Verification items for the finished model (mm, model axes). A direction names the side the tool comes from. Give positions to 0.01 mm unless a question says otherwise; leave off trailing zeros. Loops run counter-clockwise (first coordinate to the right, second up) from the corner with the lowest first, then second, coordinate; pieces in that order, holes last. Notation, with made-up numbers: (55, 60.25) - (77, 60.25) arc R18 cw to (77, 83.25) - close; hole circle Ø2 at (69, 86.25). An arc over 180 degrees is marked (long way). One line per item, written item: value. Start each with the question number.
1. Sectioned sample at C-C (z = -107.5). Record the cut outline in (x, y).
2. Gauge pin test, flat ends, axial feed: pin 1 (2 mm diameter, centred on x = 3, y = 5, fed in from -Z); pin 2 (3 mm diameter, centred on y = 2, z = -12, fed in from -X); pin 3 (1.4 mm diameter, centred on x = 2.5, y = 5.5, fed in from +Z); pin 4 (0.8 mm diameter, centred on y = 5.5, z = -126, fed in from +X). Record the tip position at first contact, or that the pin passes through.
3. Sectioned sample at B-B (x = 5.5). Record the cut outline in (y, z), plus the area to 3 significant figures.
4. Sectioned sample at A-A (y = 6.25). Record the cut outline in (x, z).
5. Mould release check, pull along Z, two halves, no side actions. Record for faces 1 (the flat face through (2, 7.302, -64)), 2 (the flat face through (3.774, 3.6, -77.998)): pulls with the +Z half, pulls with the -Z half, needs draft (parallel to the pull), parting line crosses it, or undercut.
6. Access from +Z, -Z, +X, -X, +Y, -Y to the whole of each face (thin tool, end or side, straight path). Record for faces 3 (the flat face through (1.651, 4, 1)), 4 (the flat face through (1.651, 4, -127)), 5 (the flat face through (2, 0, -64)), 6 (the flat face through (2.164, 3.6, -15.384)), 7 (the flat face through (0, 4, -64)).
7. Scan lines: L1, parallel to X at y = 5.75, z = -63.5; L2, parallel to X at y = 6.25, z = -66.5. Record each from-to range of solid material in increasing order. Write a range as [from, to].
Autodesk Inventor part; units mm, degrees
ref_plane "YZ Plane" through (0, 0, 0) normal (1, 0, 0) x (0, 1, 0)
ref_plane "XZ Plane" through (0, 0, 0) normal (0, 1, 0) x (-1, 0, 0)
ref_plane "XY Plane" through (0, 0, 0) normal (0, 0, 1) x (1, 0, 0)
sketch "Sketch1" plane through (0, 0, 0) normal (0, 1, 0) x (-1, 0, 0)
  line L0 (0, 0) -> (0, -125.2474)
  line L1 (0, -125.2474) -> (-3.4036, -125.2474)
  line L2 (0, 0) -> (-3.4036, 0)
  line L3 (-3.4036, 0) -> (-0.889, -31.2039)
  line L4 (-0.889, -31.2039) -> (-6.5786, -62.4078)
  line L5 (-6.5786, -62.4078) -> (-0.889, -94.0308)
  line L6 (-0.889, -94.0308) -> (-3.4036, -125.2474)
  dimension "d0" = 125.2474
  dimension "d1" = 3.4036
  dimension "d2" = 3.4036
  dimension "d3" = 31.2039
  dimension "d4" = 62.4078
  dimension "d5" = 31.2166
  dimension "d15" = 6.5786
  dimension "d16" = 0.889
  dimension "d17" = 0.889
extrude "Extrusion1" add sketch "Sketch1" along normal blind 7.3025
sketch "Sketch2" plane through (0, 0, 0) normal (0, 0, 1) x (1, 0, 0)
  line L0 (3.4036, 0) -> (0, 0)
  line L1 (0, 7.3025) -> (1.651, 7.3025)
  line L2 (1.651, 7.3025) -> (1.651, 0)
  line L3 (1.651, 0) -> (0, 0)
  line L4 (0, 0) -> (0, 7.3025)
  dimension "d8" = 1.651
sketch "Sketch3" plane through (3.4036, 0, -125.2474) normal (0, 0, -1) x (-1, 0, 0)
  line L0 (3.4036, 0) -> (3.4036, 7.3025)
  line L1 (0, 0) -> (3.4036, 0)
  line L2 (3.4036, 7.3025) -> (1.7526, 7.3025)
  line L3 (1.7526, 7.3025) -> (1.7526, 0)
  line L4 (1.7526, 0) -> (3.4036, 0)
  line L5 (3.4036, 0) -> (3.4036, 7.3025)
  dimension "d9" = 1.651
extrude "Extrusion2" add sketch "Sketch3" along normal blind 2.5654
extrude "Extrusion3" add sketch "Sketch2" along normal blind 2.5654
properties part number "long_insert_inv"
Results are:
1. outline: (0, 0) - (1.97, 0) - (1.97, 7.3) - (0, 7.3) - close
2. pin 1: stops at z = -125.25
2. pin 2: stops at x = 0
2. pin 3: stops at z = 0
2. pin 4: stops at x = 1.65
3. outline: (0, -68.4) - (7.3, -68.4) - (7.3, -56.49) - (0, -56.49) - close
3. area: 87.0 mm^2
4. outline: (0, -127.81) - (1.65, -127.81) - (1.65, -125.25) - (3.4, -125.25) - (0.89, -94.03) - (6.58, -62.41) - (0.89, -31.2) - (3.4, 0) - (1.65, 0) - (1.65, 2.57) - (0, 2.57) - close
5. face 1: needs draft
5. face 2: undercut
6. face 3: +Z, +X, +Y, -Y
6. face 4: -Z, +X, +Y, -Y
6. face 5: +Z, -Z, +X, -X, -Y
6. face 6: +X, +Y, -Y
6. face 7: +Z, -Z, -X, +Y, -Y
7. L1: x = [0, 6.38]
7. L2: x = [0, 5.84]
